Verification items for the finished model (mm, model axes). Face numbers are marked on the shaded views. A direction names the side the tool comes from. Coordinates: 2 decimals unless noted, no trailing zeros. Order: outer loops, then holes, each group sorted by start corner. A loop starts at its lowest first (then second) coordinate and runs counter-clockwise, first axis right, second up. Notation, with made-up numbers: M -22,2 L 22,2 A34 ccw 22,40 Z; hole C -19,36.5 d5. An arc over 180 degrees is marked long. Return JSON: item names as keys, results as strings.
```python
from build123d import *

# Parameters (mm, degrees)
ESBO_O4_R                = 3
RESSALTO_EXTRUS_O1_DEPTH = 24
CORTE_EXTRUS_O1_DEPTH    = 1.5
ESBO_O6_R                = 3.5
RESSALTO_EXTRUS_O2_DEPTH = 1
ESBO_O7_R                = 2.5
CORTE_EXTRUS_O2_DEPTH    = 1
ESBO_O8_R                = 3.25
ESBO_O8_R_2              = 3.0000000000000004
CORTE_EXTRUS_O3_DEPTH    = 0.5
FILETE2_R                = 0.5
FILETE3_R                = 1


with BuildPart() as part:
    # Esboço1 → Revolução3 (revolve)
    with BuildSketch(Plane.XY, mode=Mode.PRIVATE) as revolu_o3_sk:
        Polygon((0, 0), (4.3e-16, 4), (2.0000000000000004, 4), (2, 0), align=None)
    revolve(revolu_o3_sk.sketch.rotate(Axis((2, 0, 0), (-1, 0, 0)), 90), axis=Axis((2, 0, 0), (-1, 0, 0)))

    # Esboço4 → Ressalto-extrusão1 (add)
    with BuildSketch(Plane.ZY):
        with Locations(Location((0, 0, 0), (0, 0, 180))):
            Circle(ESBO_O4_R)
    extrude(amount=RESSALTO_EXTRUS_O1_DEPTH)

    # Esboço5 → Corte-extrusão1 (cut)
    with BuildSketch(Plane(origin=(2, 0, 0), x_dir=(0, 0, -1), z_dir=(1, 0, 0))):
        Polygon((1.3444941418500793, 2.554538869515231), (-1.5400484850299316, 2.441635516839142), (-2.88454262688001, -0.11290335267608817), (-1.3444941418500784, -2.5545388695152305), (1.540048485029931, -2.4416355168391424), (2.8845426268800107, 0.11290335267608934), align=None)
    extrude(amount=-CORTE_EXTRUS_O1_DEPTH, mode=Mode.SUBTRACT)

    # Esboço6 → Ressalto-extrusão2 (add)
    with BuildSketch(Plane.ZY.offset(24)):
        Circle(ESBO_O6_R)
    extrude(amount=RESSALTO_EXTRUS_O2_DEPTH)

    # Esboço7 → Corte-extrusão2 (cut)
    with BuildSketch(Plane.ZY.offset(25)):
        Circle(ESBO_O7_R)
    extrude(amount=-CORTE_EXTRUS_O2_DEPTH, mode=Mode.SUBTRACT)

    # Esboço8 → Corte-extrusão3 (cut)
    with BuildSketch(Plane(origin=(-24, 0, 0), x_dir=(0, 0, -1), z_dir=(1, 0, 0))):
        Circle(ESBO_O8_R)
        Circle(ESBO_O8_R_2, mode=Mode.SUBTRACT)
    extrude(amount=-CORTE_EXTRUS_O3_DEPTH, mode=Mode.SUBTRACT)

    # Filete2
    # the kernel refuses this fillet: 0.5 mm, written as the material it adds along each edge
    with BuildSketch(Plane(origin=(-24, 0, 0), x_dir=(0, 0, 1), z_dir=(0, -1, 0))) as filete2_piece_1:
        with BuildLine():
            CenterArc((2.5 - FILETE2_R, FILETE2_R), FILETE2_R, 270, 90)
            Line((2.5 - FILETE2_R, 0), (2.5 - FILETE2_R, -FILETE2_R * 0.02))
            Line((2.5 - FILETE2_R, -FILETE2_R * 0.02), (2.5 + FILETE2_R * 0.02, -FILETE2_R * 0.02))
            Line((2.5 + FILETE2_R * 0.02, -FILETE2_R * 0.02), (2.5 + FILETE2_R * 0.02, FILETE2_R))
            Line((2.5 + FILETE2_R * 0.02, FILETE2_R), (2.5, FILETE2_R))
        make_face()
    revolve(axis=Axis((-24, 0, 0), (-1, 0, 0)))
    with BuildSketch(Plane(origin=(-24.5, 0, 0), x_dir=(0, 0, -1), z_dir=(0, -1, 0))) as filete2_piece_2:
        with BuildLine():
            CenterArc((3.5000000000000004, 0.4330127018922383), FILETE2_R, 180, 60.00000000000102)
            Line((3.0000000000000004, 0.4330127018922383), (2.9900000000000007, 0.4330127018922383))
            Line((2.9900000000000007, 0.4330127018922383), (2.9900000000000007, 0))
            Line((2.9900000000000007, 0), (3.0000000000000004, -0.01000000000000156))
            ThreePointArc((3.0000000000000004, -0.01000000000000156), (3.1250000000000044, -0.01000000000000156), (3.2450000000000085, -0.00866025403783155))
            Line((3.2450000000000085, -0.00866025403783155), (3.2500000000000084, 1.421e-14))
        make_face()
    revolve(axis=Axis((-24.5, 0, 0), (1, 0, 0)))
    with BuildSketch(Plane(origin=(0, 0, 0), x_dir=(0, 1.2e-16, -1), z_dir=(0, 1, 1.2e-16))) as filete2_piece_3:
        with BuildLine():
            CenterArc((3 + FILETE2_R, FILETE2_R), FILETE2_R, 180, 90)
            Line((3 + FILETE2_R, -6e-17), (3 + FILETE2_R, -FILETE2_R * 0.02))
            Line((3 + FILETE2_R, -FILETE2_R * 0.02), (3 - FILETE2_R * 0.02, -FILETE2_R * 0.02))
            Line((3 - FILETE2_R * 0.02, -FILETE2_R * 0.02), (3 - FILETE2_R * 0.02, FILETE2_R))
            Line((3 - FILETE2_R * 0.02, FILETE2_R), (3, FILETE2_R))
        make_face()
    revolve(axis=Axis((0, 0, 0), (-1, 0, 0)))
    # the kernel refuses this fillet: 0.5 mm, written as the material it takes off along each edge
    with BuildSketch(Plane(origin=(-25, 0, 0), x_dir=(0, 0, 1), z_dir=(0, -1, 0))) as filete2_2_piece_1:
        with BuildLine():
            CenterArc((3.5 - FILETE2_R, -FILETE2_R), FILETE2_R, 0, 90)
            Line((3.5 - FILETE2_R, 0), (3.5 - FILETE2_R, FILETE2_R * 0.02))
            Line((3.5 - FILETE2_R, FILETE2_R * 0.02), (3.5 + FILETE2_R * 0.02, FILETE2_R * 0.02))
            Line((3.5 + FILETE2_R * 0.02, FILETE2_R * 0.02), (3.5 + FILETE2_R * 0.02, -FILETE2_R))
            Line((3.5 + FILETE2_R * 0.02, -FILETE2_R), (3.5, -FILETE2_R))
        make_face()
    revolve(axis=Axis((-25, 0, 0), (-1, 0, 0)), mode=Mode.SUBTRACT)
    with BuildSketch(Plane(origin=(-24, 0, 0), x_dir=(0, 0, -1), z_dir=(0, -1, 0))) as filete2_2_piece_2:
        with BuildLine():
            CenterArc((3.75, -0.4330127018922454), FILETE2_R, 119.99999999999864, 60.000000000001364)
            Line((3.25, -0.4330127018922454), (3.24, -0.4330127018922454))
            Line((3.24, -0.4330127018922454), (3.24, 0))
            Line((3.24, 0), (3.25, 0.01000000000000156))
            ThreePointArc((3.25, 0.01000000000000156), (3.3750000000000053, 0.01000000000000156), (3.495000000000011, 0.00866025403782444))
            Line((3.495000000000011, 0.00866025403782444), (3.500000000000011, -2.132e-14))
        make_face()
    revolve(axis=Axis((-24, 0, 0), (1, 0, 0)), mode=Mode.SUBTRACT)

    # Filete3
    filete3_edges = [part.edges().sort_by_distance(p)[0] for p in [
        (0.5, 1.3337211110956604, -2.114518384365045),
        (0.5, -1.1643660820815265, -2.212295555954971),
        (0.5, -2.498087193177186, -0.09777717158992649),
        (0.5, -1.3337211110956593, 2.114518384365044),
        (0.5, 1.164366082081527, 2.212295555954971),
        (0.5, 2.498087193177186, 0.09777717158992627),
    ]]
    fillet(filete3_edges, radius=FILETE3_R)


solid = part.part
```
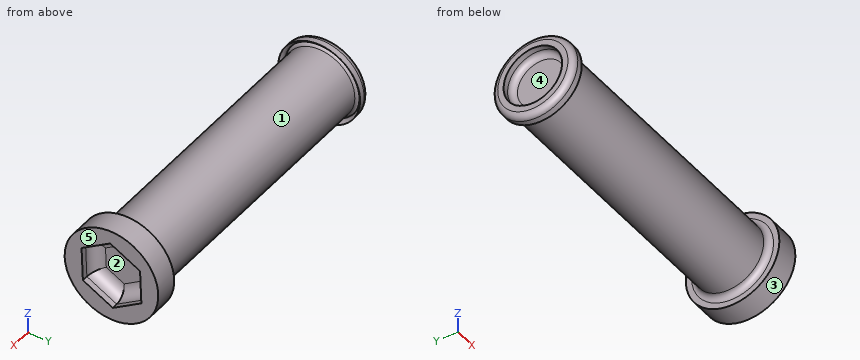
Q1. Cross-section at A-A, the plane x = -21.75. Record the boundary of the cut face in (y, z), and give its area (3 significant figures).
Values:
{"outline": "C 0,0 d6", "area": "28.3 mm^2"}
Q2. Material ranges on line 1 along X through (y, z) = (1.5, 1); line 2 along X through (y, z) = (2.5, -2.5); line 3 along Y through (x, z) = (-12.5, -1.75), recorded low to high.
Values:
{"line 1": "-24 to 0.5", "line 2": "0 to 2", "line 3": "-2.44 to 2.44"}
Q3. Go/stop test with flat-tipped pins: pin 1 (4 mm diameter, centred on x = -10, y = -1.5, fed in from +Z); pin 2 (1.5 mm diameter, centred on x = -16.5, y = -2.5, fed in from +Z); pin 3 (1.5 mm diameter, centred on x = -6.5, z = -1.5, fed in from +Y). Record where each tip stops, or that it passes through.
Values:
{"pin 1": "z = 3", "pin 2": "z = 2.44", "pin 3": "y = 2.9"}
Q4. Tool access check on the marked faces 1 and 2. Record the directions out of +Z, -Z, +X, -X, +Y, -Y that give a thin tool (end or side, any length) a straight path to the whole face; none if there is none.
Values:
{"face 1": "none", "face 2": "+X"}
Q5. Draft check along Y on the marked faces 3, 4 and 5. Enter one of: pulls with the +Y half, pulls with the -Y half, needs draft (parallel to the pull), parting line crosses it, or undercut.
Values:
{"face 3": "parting line crosses it", "face 4": "undercut", "face 5": "needs draft"}
